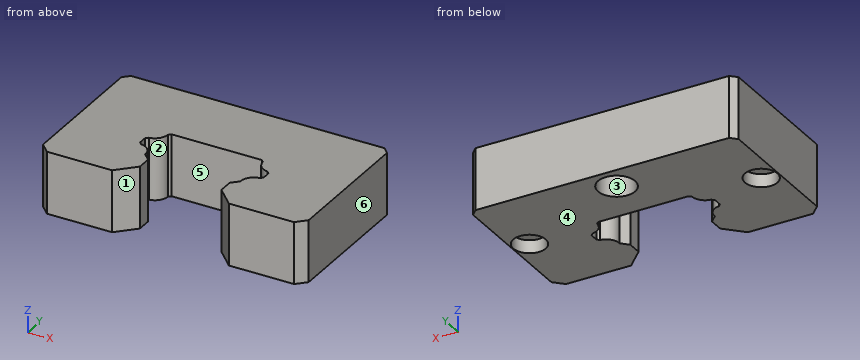
Autodesk Inventor part; units mm, degrees
ref_plane "YZ Plane" through (0, 0, 0) normal (1, 0, 0) x (0, 1, 0)
ref_plane "XZ Plane" through (0, 0, 0) normal (0, 1, 0) x (-1, 0, 0)
ref_plane "XY Plane" through (0, 0, 0) normal (0, 0, 1) x (1, 0, 0)
sketch "Sketch1" plane through (0, 0, 0) normal (0, 0, 1) x (1, 0, 0)
  line L0 (20.5165, 15) -> (21.5, 14.0165)
  line L1 (-20.5165, 15) -> (20.5165, 15)
  line L2 (-21.5, 14.0165) -> (-20.5165, 15)
  line L3 (-21.5, -8) -> (-21.5, 14.0165)
  line L4 (-20, -9.5) -> (-21.5, -8)
  line L5 (-9.45, -9.5) -> (-20, -9.5)
  line L6 (-6.6, -6.65) -> (-9.45, -9.5)
  line L7 (-6.6, -4.35) -> (-6.6, -6.65)
  line L8 (-7.7, -3.25) -> (-6.6, -4.35)
  arc A0 (-7.7, -3.25) -> (-9.6, -1.075) centre (-9.8292, -3.1926) ccw
  line L9 (-10, -0.675) -> (-9.6, -1.075)
  line L10 (-10, 0.675) -> (-10, -0.675)
  line L11 (-9.6, 1.075) -> (-10, 0.675)
  arc A1 (-9.6, 1.075) -> (-7.7, 3.1) centre (-9.828, 3.1928) ccw
  line L12 (-7.3, 3.5) -> (-7.7, 3.1)
  line L13 (7.3, 3.5) -> (-7.3, 3.5)
  line L14 (7.7, 3.1) -> (7.3, 3.5)
  arc A2 (7.7, 3.1) -> (9.6, 1.075) centre (9.828, 3.1928) ccw
  line L15 (10, 0.675) -> (9.6, 1.075)
  line L16 (10, -0.675) -> (10, 0.675)
  line L17 (9.6, -1.075) -> (10, -0.675)
  arc A3 (9.6, -1.075) -> (7.7, -3.25) centre (9.8292, -3.1926) ccw
  line L18 (6.6, -4.35) -> (7.7, -3.25)
  line L19 (6.6, -6.65) -> (6.6, -4.35)
  line L20 (9.45, -9.5) -> (6.6, -6.65)
  line L21 (20, -9.5) -> (9.45, -9.5)
  line L22 (21.5, -8) -> (20, -9.5)
  line L23 (21.5, 14.0165) -> (21.5, -8)
  circle A4 centre (-18.75, 2.9) radius 2.625
  circle A5 centre (18.75, 2.9) radius 2.625
  point P0 (0, 0)
  point P1 (0, 0)
extrude "Extrusion1" add sketch "Sketch1" along normal blind 10 contours L0 L23 L22 L21 L20 L19 L18 A3 L17 L16 L15 A2 L14 L13 L12 A1 L11 L10 L9 A0 L8 L7 L6 L5 L4 L3 L2 L1 | A4 | A5
extrude "Extrusion2" cut sketch "Sketch1" along normal blind 2.1 contours A4 | A5
sketch "Sketch2" plane through (0, 0, 0) normal (0, 0, -1) x (-1, 0, 0)
  circle A0 centre (18.75, 2.9) radius 2.625
  circle A1 centre (-18.75, 2.9) radius 2.625
  line L0 (-7.7, -3.25) -> (-6.6, -4.35)
  arc A2 (-7.7, -3.25) -> (-9.6, -1.075) centre (-9.8292, -3.1926) ccw
  line L1 (-10, -0.675) -> (-9.6, -1.075)
  line L2 (-10, 0.675) -> (-10, -0.675)
  line L3 (-9.6, 1.075) -> (-10, 0.675)
  arc A3 (-9.6, 1.075) -> (-7.7, 3.1) centre (-9.828, 3.1928) ccw
  line L4 (-7.3, 3.5) -> (-7.7, 3.1)
  line L5 (7.3, 3.5) -> (-7.3, 3.5)
  line L6 (7.7, 3.1) -> (7.3, 3.5)
  arc A4 (7.7, 3.1) -> (9.6, 1.075) centre (9.828, 3.1928) ccw
  line L7 (10, 0.675) -> (9.6, 1.075)
  line L8 (10, -0.675) -> (10, 0.675)
  line L9 (9.6, -1.075) -> (10, -0.675)
  arc A5 (9.6, -1.075) -> (7.7, -3.25) centre (9.8292, -3.1926) ccw
  line L10 (6.6, -4.35) -> (7.7, -3.25)
  line L11 (6.6, -6.65) -> (6.6, -4.35)
  line L12 (9.45, -9.5) -> (6.6, -6.65)
  line L13 (20, -9.5) -> (9.45, -9.5)
  line L14 (21.5, -8) -> (20, -9.5)
  line L15 (21.5, 14.0165) -> (21.5, -8)
  line L16 (20.5165, 15) -> (21.5, 14.0165)
  line L17 (-20.5165, 15) -> (20.5165, 15)
  line L18 (-21.5, 14.0165) -> (-20.5165, 15)
  line L19 (-21.5, -8) -> (-21.5, 14.0165)
  line L20 (-20, -9.5) -> (-21.5, -8)
  line L21 (-9.45, -9.5) -> (-20, -9.5)
  line L22 (-6.6, -6.65) -> (-9.45, -9.5)
  line L23 (-6.6, -4.35) -> (-6.6, -6.65)
  circle A6 centre (0, 11) radius 3
  point P0 (0, 0)
  point P1 (0, 0)
extrude "Extrusion3" cut sketch "Sketch2" against normal blind 4 contours A6
properties part number "HGR20C"
The listing builds one solid part. Answer for the finished solid, in the listing's coordinates (mm). Face numbers are marked on the shaded views. A direction names the side the tool comes from. Round coordinates to 2 decimals unless told otherwise and drop trailing zeros. Loops run counter-clockwise (first coordinate to the right, second up) from the corner with the lowest first, then second, coordinate; pieces in that order, holes last.
Q1. Section D-D, the plane y = 11 is taken. Determine the outline of the cut face in (x, z), then the cut area to 3 significant figures.
Q2. Find the intervals of material crossed by line 1 (Y direction, x = 0, z = 2.2); line 2 (Y direction, x = 18.75, z = 1.6) (3 decimals); line 3 (X direction, y = -3, z = 4.75), in increasing order.
Q3. Section C-C, the plane y = -2.25 is taken. Determine the outline of the cut face in (x, z).
Q4. Given pin 1 Ø1.6 at (x, y) = (18.5, 4) entering from -Z; pin 2 Ø6 at (x, z) = (0, 8.5) entering from -Y; pin 3 Ø5.5 at (x, y) = (0, 11) entering from -Z, each flat-ended and moving along its own axis, determine where each tip first touches the part or whether it passes through.
Q5. For a pull along X with two mould halves and no side action, classify the marked faces 4, 5 and 6 as released by +X, released by -X, zero draft, split by the parting line, or undercut.
Q6. Which of the six approach directions +Z, -Z, +X, -X, +Y, -Y give full straight-line access (tool end or side, diameter ignored) to the marked faces 1, 2 and 3?
Q7. Section B-B, the plane x = -18.75 is taken. Determine the outline of the cut face in (y, z) (3 decimals).
Completed:
1. outline: (-21.5, 0) - (-3, 0) - (-3, 4) - (3, 4) - (3, 0) - (21.5, 0) - (21.5, 10) - (-21.5, 10) - close
1. area: 406 mm2
2. line 1: y = 3.5 to 8, 14 to 15
2. line 2: y = -9.5 to 0.275, 5.525 to 15
2. line 3: x = -21.5 to -7.71, 7.71 to 21.5
3. outline: (-21.5, 0) - (-7.92, 0) - (-7.92, 10) - (-21.5, 10) - close; (7.92, 0) - (21.5, 0) - (21.5, 10) - (7.92, 10) - close
4. pin 1: stops at z = 2.1
4. pin 2: stops at y = 3.5
4. pin 3: stops at z = 4
5. face 4: zero draft
5. face 5: undercut
5. face 6: released by +X
6. face 1: +Z, -Z, -Y
6. face 2: +Z, -Z
6. face 3: -Z
7. outline: (-9.5, 0) - (0.275, 0) - (0.275, 2.1) - (5.525, 2.1) - (5.525, 0) - (15, 0) - (15, 10) - (-9.5, 10) - close
